```python
from build123d import *

# Parameters (mm, degrees)
ESBO_O1_R                = 15.995
RESSALTO_EXTRUS_O1_DEPTH = 33.35
ESBO_O2_R                = 26.91
RESSALTO_EXTRUS_O2_DEPTH = 8.1
ESBO_O3_R                = 4.61
CORTE_EXTRUS_O1_DEPTH    = 5
ESBO_O4_R                = 2.755
CORTE_EXTRUS_O2_DEPTH    = 8.1
ESBO_O5_R                = 10.2
CORTE_EXTRUS_O3_DEPTH    = 41.45


with BuildPart() as part:
    # Esboço1 → Ressalto-extrusão1 (new body)
    with BuildSketch(Plane.XY):
        Circle(ESBO_O1_R)
    extrude(amount=RESSALTO_EXTRUS_O1_DEPTH)

    # Esboço2 → Ressalto-extrusão2 (add)
    with BuildSketch(Plane.XY.offset(33.35)):
        Circle(ESBO_O2_R)
    extrude(amount=RESSALTO_EXTRUS_O2_DEPTH)

    # Esboço3 → Corte-extrusão1 (cut)
    with BuildSketch(Plane.XY.offset(41.45)):
        with Locations((21.45, 0)):
            Circle(ESBO_O3_R)
        with Locations((0, -21.45)):
            Circle(ESBO_O3_R)
        with Locations((-21.45, 0)):
            Circle(ESBO_O3_R)
        with Locations((0, 21.45)):
            Circle(ESBO_O3_R)
    extrude(amount=-CORTE_EXTRUS_O1_DEPTH, mode=Mode.SUBTRACT)

    # Esboço4 → Corte-extrusão2 (cut)
    with BuildSketch(Plane.XY.offset(41.45)):
        with Locations((21.45, 0)):
            Circle(ESBO_O4_R)
        with Locations((0, -21.45)):
            Circle(ESBO_O4_R)
        with Locations((-21.45, 0)):
            Circle(ESBO_O4_R)
        with Locations((0, 21.45)):
            Circle(ESBO_O4_R)
    extrude(amount=-CORTE_EXTRUS_O2_DEPTH, mode=Mode.SUBTRACT)

    # Esboço5 → Corte-extrusão3 (cut)
    with BuildSketch(Plane.XY.offset(41.45)):
        Circle(ESBO_O5_R)
    extrude(amount=-CORTE_EXTRUS_O3_DEPTH, mode=Mode.SUBTRACT)


solid = part.part
```
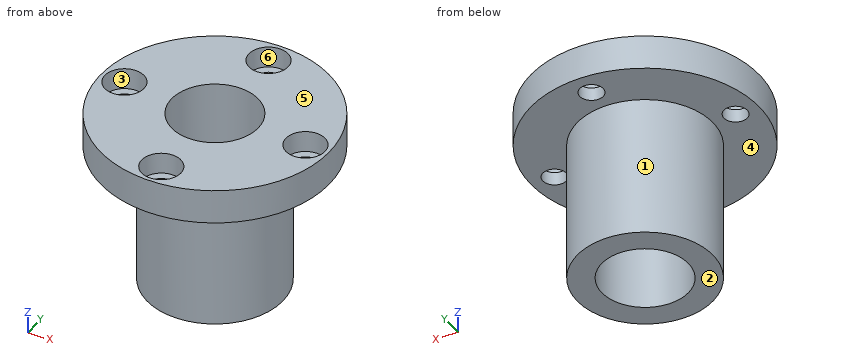
Geometry: final body of the model. Coordinates: model frame, mm. Face numbers are marked on the shaded views. A direction names the side the tool comes from. Round coordinates to 2 decimals unless told otherwise and drop trailing zeros. Loops run counter-clockwise (first coordinate to the right, second up) from the corner with the lowest first, then second, coordinate; pieces in that order, holes last. Notation, with made-up numbers: (-13, 89) -> (15, 89) arc R25 ccw to (15, 115) -> close; hole circle Ø6 at (-18, -31). An arc over 180 degrees is marked (long way). Use one line per item in the form item = value. Start each with the question number.
1) Line query: L1, parallel to Y at x = 0, z = 39; L2, parallel to Y at x = -1.5, z = 34.5; L3, parallel to Z at x = 23, y = 6.5. Output: solid intervals per line, ascending.
2) Section C-C on y = 6.5. Output: boundary loops of the cut face in (x, z), then the cut area to 3 significant figures.
3) Section D-D on z = 37.5. Output: boundary loops of the cut face in (x, y), then the cut area to 3 significant figures.
4) Section A-A on x = 0. Output: boundary loops of the cut face in (y, z) (3 decimals), then the cut area to 3 significant figures.
5) Access query for the marked faces 4, 5 and 6. Directions: +Z, -Z, +X, -X, +Y, -Y. A direction counts if a zero-diameter tool reaches every point of the face in a straight line with its end or side. Return the directions, or none.
6) Draft query along Y for the marked faces 1, 2 and 3. Return one class per face: released by +Y, released by -Y, zero draft, split by the parting line, or undercut.
7) First-contact query: P1, Ø7, axis at x = 0, y = -21.45, coming from the -Z side; P2, Ø4, axis at x = -3, z = 29, coming from the +Y side; P3, Ø3, axis at x = 9.5, z = 36.5, coming from the +Y side; P4, Ø10, axis at x = 0.5, y = 22.5, coming from the +Z side. Flat tips, straight axial feed; report the tip coordinate or a pass-through.
Response:
q1.L1 = -26.91 to -26.06, -16.84 to -10.2, 10.2 to 16.84, 26.06 to 26.91
q1.L2 = -26.87 to -23.76, -19.14 to -10.09, 10.09 to 19.14, 23.76 to 26.87
q1.L3 = 33.35 to 41.45
q2.outline = (-26.11, 33.35) -> (-14.61, 33.35) -> (-14.61, 0) -> (-7.86, 0) -> (-7.86, 41.45) -> (-26.11, 41.45) -> close; (7.86, 0) -> (14.61, 0) -> (14.61, 33.35) -> (26.11, 33.35) -> (26.11, 41.45) -> (7.86, 41.45) -> close
q2.area = 746 mm^2
q3.outline = circle Ø53.82 at (0, 0); hole circle Ø9.22 at (-21.45, 0); hole circle Ø20.4 at (0, 0); hole circle Ø9.22 at (0, -21.45); hole circle Ø9.22 at (0, 21.45); hole circle Ø9.22 at (21.45, 0)
q3.area = 1,680 mm^2
q4.outline = (-26.91, 33.35) -> (-24.205, 33.35) -> (-24.205, 36.45) -> (-26.06, 36.45) -> (-26.06, 41.45) -> (-26.91, 41.45) -> close; (-18.695, 33.35) -> (-15.995, 33.35) -> (-15.995, 0) -> (-10.2, 0) -> (-10.2, 41.45) -> (-16.84, 41.45) -> (-16.84, 36.45) -> (-18.695, 36.45) -> close; (10.2, 0) -> (15.995, 0) -> (15.995, 33.35) -> (18.695, 33.35) -> (18.695, 36.45) -> (16.84, 36.45) -> (16.84, 41.45) -> (10.2, 41.45) -> close; (24.205, 33.35) -> (26.91, 33.35) -> (26.91, 41.45) -> (26.06, 41.45) -> (26.06, 36.45) -> (24.205, 36.45) -> close
q4.area = 531 mm^2
q5.face_4 = -Z
q5.face_5 = +Z, +X, -X, +Y, -Y
q5.face_6 = +Z
q6.face_1 = split by the parting line
q6.face_2 = zero draft
q6.face_3 = undercut
q7.P1 = 33.35
q7.P2 = 15.96
q7.P3 = 25.69
q7.P4 = 41.45
